Model file for the job. Use its own axes, mm. Face numbers are marked on the shaded views. A direction names the side the tool comes from. Round coordinates to 2 decimals unless told otherwise and drop trailing zeros. Loops run counter-clockwise (first coordinate to the right, second up) from the corner with the lowest first, then second, coordinate; pieces in that order, holes last. Notation, with made-up numbers: M -19.5,65.5 L 28.5,65.5 A14 cw 28.5,73.5 Z; hole C 68,81.5 d7. An arc over 180 degrees is marked long. Answer in a Markdown table with one row per item.
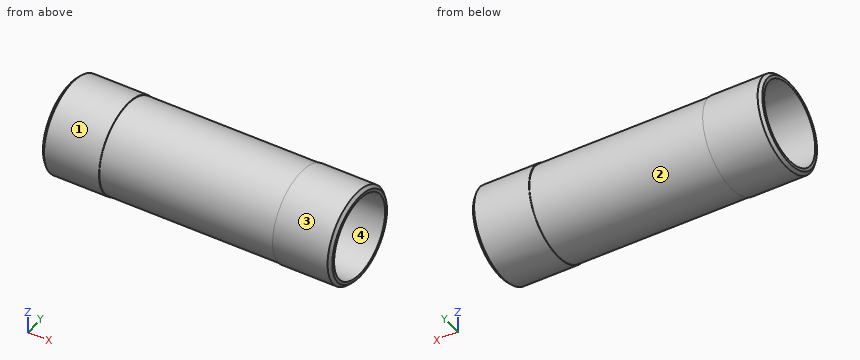
Autodesk Inventor part; units mm, degrees
ref_plane "YZ Plane" through (0, 0, 0) normal (1, 0, 0) x (0, 1, 0)
ref_plane "XZ Plane" through (0, 0, 0) normal (0, 1, 0) x (-1, 0, 0)
ref_plane "XY Plane" through (0, 0, 0) normal (0, 0, 1) x (1, 0, 0)
sketch "Skizze1" plane through (0, 0, 0) normal (0, 0, 1) x (1, 0, 0)
  line L0 (-60, 0) -> (10, 0)
  line L1 (0, -1.6) -> (0, 9.6)
  line L2 (0, 7) -> (-50, 7)
  line L3 (-50, 7) -> (-50, 8)
  line L4 (-50, 8) -> (-40, 8)
  line L5 (-40, 8) -> (-40, 7.9)
  line L6 (-40, 7.9) -> (-10, 7.9)
  line L7 (-10, 7.9) -> (-10, 8)
  line L8 (-10, 8) -> (0, 8)
  line L9 (0, 7) -> (0, 8)
  point P0 (0, 0)
  dimension "d1" = 14
  dimension "d2" = 16
  dimension "d4" = 50
  dimension "d5" = 10
  dimension "d6" = 10
  dimension "d11" = 0.1
revolve "Umdrehung1" add sketch "Skizze1" angle 360 about axis through (-10, 0, 0) along (1, 0, 0)
chamfer "Fase1" distance 0.5 angle 45 2 edges at (0, -8, 0) (-50, -8, 0)
properties part number "13_0204_033"
1. Wall check: probe 1 along Z at (x, y) = (-12, 0); probe 2 along Y at (x, z) = (-46.5, 5.25); probe 3 along Z at (x, y) = (-4, 1.5). Give the ranges that are in metal, low to high.
Verdict:
| item | result |
|---|---|
| probe 1 | z = -7.9 to -7, 7 to 7.9 |
| probe 2 | y = -6.04 to -4.63, 4.63 to 6.04 |
| probe 3 | z = -7.86 to -6.84, 6.84 to 7.86 |
2. Saw through at D-D (x = -18). Write the cut outline in (y, z).
Verdict:
| item | result |
|---|---|
| outline | C 0,0 d15.8; hole C 0,0 d14 |
3. Mould opens along Y. For the marked faces 3 and 4 say: +Y half, -Y half, draft (parallel to the pull), parting line (faces both ways), or undercut.
Verdict:
| item | result |
|---|---|
| face 3 | parting line |
| face 4 | undercut |
4. Saw through at A-A (y = 0). Write the cut outline in (x, z), and give its area (3 significant figures).
Verdict:
| item | result |
|---|---|
| outline | M -50,-7.5 L -49.5,-8 L -40,-8 L -40,-7.9 L -10,-7.9 L -10,-8 L -0.5,-8 L 0,-7.5 L 0,-7 L -50,-7 Z; M -50,7 L 0,7 L 0,7.5 L -0.5,8 L -10,8 L -10,7.9 L -40,7.9 L -40,8 L -49.5,8 L -50,7.5 Z |
| area | 93.5 mm² |
5. Tool access for the marked faces 1 and 2: list every direction of +Z, -Z, +X, -X, +Y, -Y with a clear straight run to the whole face (end or side of a thin tool).
Verdict:
| item | result |
|---|---|
| face 1 | +X, -X |
| face 2 | none |
6. Saw through at C-C (x = -9.5). Write the cut outline in (y, z).
Verdict:
| item | result |
|---|---|
| outline | C 0,0 d16; hole C 0,0 d14 |
7. Pin check, flat tips, straight feed: pin 1 (4 mm diameter, centred on x = -26, z = 1.5, fed in from -Y); pin 2 (6 mm diameter, centred on x = -39, z = -4, fed in from +Y); pin 3 (4 mm diameter, centred on x = -13.5, y = -2, fed in from -Z). Stop position of each tip, or through.
Verdict:
| item | result |
|---|---|
| pin 1 | stops at y = -7.9 |
| pin 2 | stops at y = 7.91 |
| pin 3 | stops at z = -7.9 |
